```python
from build123d import *

# Parameters (mm, degrees)
SKETCH_1_W           = 30
SKETCH_1_H           = 48
EXTRUDE_1_DEPTH      = 2
SKETCH_2_R           = 1.6
CUT_EXTRUDE_1_DEPTH  = 2
SKETCH_3_R           = 8.75
CUT_EXTRUDE_2_DEPTH  = 2
SKETCH_4_W           = 30
SKETCH_4_H           = 2
EXTRUDE_2_DEPTH      = 17
SKETCH_14_W          = 0.5
SKETCH_14_H          = 2
CUT_EXTRUDE_6_DEPTH  = 67.738294854
SKETCH_15_W          = 2
SKETCH_15_H          = 65
EXTRUDE_7_DEPTH      = 50
SKETCH_16_W          = 5
SKETCH_16_H          = 65
EXTRUDE_8_DEPTH      = 35
SKETCH_17_R          = 2
CUT_EXTRUDE_7_DEPTH  = 35
SKETCH_18_W          = 2
SKETCH_18_H          = 28.264297395
EXTRUDE_9_DEPTH      = 1
EXTRUDE_10_REACH     = 87.675
SKETCH_19_W          = 2
SKETCH_19_H          = 19.264297395
CUT_EXTRUDE_8_DEPTH  = 6
CUT_EXTRUDE_9_DEPTH  = 6
CHAMFER_1_SIZE       = 1.5
SKETCH_22_R          = 1.5
SKETCH_22_W          = 4
SKETCH_22_H          = 11
CUT_EXTRUDE_10_DEPTH = 86.293610546


with BuildPart() as part:
    # Sketch 1 → Extrude 1 (new body)
    with BuildSketch(Plane.XY):
        Rectangle(SKETCH_1_W, SKETCH_1_H)
    extrude(amount=-EXTRUDE_1_DEPTH)

    # Sketch 2 → Cut-Extrude 1 (cut)
    with BuildSketch(Plane.XY):
        with Locations((-9.5, 19)):
            Circle(SKETCH_2_R)
        with Locations((9.5, 19)):
            Circle(SKETCH_2_R)
    extrude(amount=-CUT_EXTRUDE_1_DEPTH, mode=Mode.SUBTRACT)

    # Sketch 3 → Cut-Extrude 2 (cut)
    with BuildSketch(Plane.XY):
        with Locations((0, 13)):
            Circle(SKETCH_3_R)
    extrude(amount=-CUT_EXTRUDE_2_DEPTH, mode=Mode.SUBTRACT)

    # Sketch 4 → Extrude 2 (add)
    with BuildSketch(Plane(origin=(0, 24, 0), x_dir=(1, 0, 0), z_dir=(0, 1, 0))):
        with Locations((0, 1)):
            Rectangle(SKETCH_4_W, SKETCH_4_H)
    extrude(amount=EXTRUDE_2_DEPTH)

    # Sketch 14 → Cut-Extrude 6 (cut, through all)
    with BuildSketch(Plane.XZ.offset(24)):
        with Locations((-0.25, -1)):
            Rectangle(SKETCH_14_W, SKETCH_14_H)
    extrude(amount=-CUT_EXTRUDE_6_DEPTH, mode=Mode.SUBTRACT)


with BuildPart() as cut_extrude_6_piece_1:
    # of the separate pieces the step leaves, piece 1, a body of its own (cut_extrude_6_pieces)
    add(part.part.solids().sort_by_distance((15, -24, 0))[0])

    # Sketch 15 → Extrude 7 (add)
    with BuildSketch(Plane(origin=(15, 0, 0), x_dir=(0, 0, -1), z_dir=(1, 0, 0))):
        with Locations((1, 8.5)):
            Rectangle(SKETCH_15_W, SKETCH_15_H)
    extrude(amount=EXTRUDE_7_DEPTH)

    # Sketch 16 → Extrude 8 (add)
    with BuildSketch(Plane(origin=(0, 0, -2), x_dir=(-1, 0, 0), z_dir=(0, 0, -1))):
        with Locations((-62.5, 8.5)):
            Rectangle(SKETCH_16_W, SKETCH_16_H)
    extrude(amount=EXTRUDE_8_DEPTH)

    # Sketch 17 → Cut-Extrude 7 (cut)
    with BuildSketch(Plane(origin=(65, 0, 0), x_dir=(0, 0, -1), z_dir=(1, 0, 0))):
        with Locations(Location((13.5, 8.5, 0), (0, 0, 90))):
            Circle(SKETCH_17_R)
        with Locations(Location((23.5, 8.5, 0), (0, 0, 90))):
            Circle(SKETCH_17_R)
    extrude(amount=-CUT_EXTRUDE_7_DEPTH, mode=Mode.SUBTRACT)



with BuildPart() as cut_extrude_6_piece_2:
    # of the separate pieces the step leaves, piece 2, a body of its own (cut_extrude_6_pieces)
    add(part.part.solids().sort_by_distance((-15, -24, 0))[0])


with BuildPart() as cut_extrude_6_piece_1_1:
    add(cut_extrude_6_piece_1.part)

    add(cut_extrude_6_piece_2.part)  # Extrude 9 merges Cut-Extrude 6 piece 2
    # Sketch 18 → Extrude 9 (add)
    with BuildSketch(Plane(origin=(-0.5, 0, 0), x_dir=(0, 0, -1), z_dir=(1, 0, 0))):
        with Locations((1, -9.867851303)):
            Rectangle(SKETCH_18_W, SKETCH_18_H)
    extrude(amount=EXTRUDE_9_DEPTH)

    # Sketch 19 → Extrude 10 (add, up to next)
    with BuildSketch(Plane(origin=(-0.5, 0, 0), x_dir=(0, 0, -1), z_dir=(1, 0, 0)), mode=Mode.PRIVATE) as extrude_10_sk1:
        with Locations((1, 31.367851303)):
            Rectangle(SKETCH_19_W, SKETCH_19_H)
    extrude_10_tool1 = extrude(extrude_10_sk1.sketch, amount=EXTRUDE_10_REACH, mode=Mode.PRIVATE) - cut_extrude_6_piece_1_1.part
    add(extrude_10_tool1.solids().sort_by_distance((-0.5, 31.367851, -1))[0])

    # Sketch 20 → Cut-Extrude 8 (cut)
    with BuildSketch(Plane.XY):
        with BuildLine():
            Line((30, -5.5), (55, -5.5))
            ThreePointArc((55, -5.5), (58.5, -9), (55, -12.5))
            Line((55, -12.5), (30, -12.5))
            ThreePointArc((30, -12.5), (26.5, -9), (30, -5.5))
        make_face()
    extrude(amount=-CUT_EXTRUDE_8_DEPTH, mode=Mode.SUBTRACT)

    # Sketch 21 → Cut-Extrude 9 (cut)
    with BuildSketch(Plane(origin=(65, 0, 0), x_dir=(0, 0, -1), z_dir=(1, 0, 0))):
        with BuildLine():
            Line((7, -11), (32, -11))
            ThreePointArc((32, -11), (35, -14), (32, -17))
            Line((32, -17), (7, -17))
            ThreePointArc((7, -17), (4, -14), (7, -11))
        make_face()
    extrude(amount=-CUT_EXTRUDE_9_DEPTH, mode=Mode.SUBTRACT)

    # Chamfer 1
    chamfer_1_edges = [cut_extrude_6_piece_1_1.edges().sort_by_distance(p)[0] for p in [
        (60, 8.5, -2),
    ]]
    chamfer(chamfer_1_edges, length=CHAMFER_1_SIZE - 0.0001)  # a hair under: the kernel refuses the full size

    # Sketch 22 → Cut-Extrude 10 (cut, through all)
    with BuildSketch(Plane.XY):
        with Locations((-5, 38)):
            Circle(SKETCH_22_R)
        with Locations((-5, 27)):
            Circle(SKETCH_22_R)
        with Locations((7, 32.5)):
            Rectangle(SKETCH_22_W, SKETCH_22_H)
    extrude(amount=-CUT_EXTRUDE_10_DEPTH, mode=Mode.SUBTRACT)


solid = cut_extrude_6_piece_1_1.part
```
Work out the finished part from the listing and answer in its coordinate system (mm). A direction names the side the tool comes from. Round coordinates to 2 decimals unless told otherwise and drop trailing zeros. Loops run counter-clockwise (first coordinate to the right, second up) from the corner with the lowest first, then second, coordinate; pieces in that order, holes last.
(1) The part is cut by section A-A, the plane z = -18. Give the vertices of the cut face in (x, y), and give its area (3 significant figures).
Computed values:
outline: (60, -24) - (65, -24) - (65, -17) - (60, -17) - close; (60, -11) - (65, -11) - (65, 41) - (60, 41) - close
area: 295 mm2
(2) Find the intervals of material crossed by L1, parallel to Z at x = 63, y = 8; L2, parallel to Z at x = 63.25, y = 8.5; L3, parallel to X at y = 12, z = -25, in increasing order.
Computed values:
L1: z = -37 to -25.44, -21.56 to -15.44, -11.56 to 0
L2: z = -37 to -25.5, -21.5 to -15.5, -11.5 to 0
L3: x = 60 to 65
(3) The part is cut by section C-C, the plane z = -23.5. Give the vertices of the cut face in (x, y).
Computed values:
outline: (60, -24) - (65, -24) - (65, -17) - (60, -17) - close; (60, -11) - (65, -11) - (65, 6.5) - (60, 6.5) - close; (60, 10.5) - (65, 10.5) - (65, 41) - (60, 41) - close
(4) The part is cut by section B-B, the plane x = 38. Give the vertices of the cut face in (y, z), and give its area (3 significant figures).
Computed values:
outline: (-24, -2) - (-12.5, -2) - (-12.5, 0) - (-24, 0) - close; (-5.5, -2) - (41, -2) - (41, 0) - (-5.5, 0) - close
area: 116 mm2
(5) For faces 1 (the cylindrical face through (63, -14, -35)), 2 (the flat face through (-15, 8, -1)), 3 (the flat face through (63, 9, -37)), 4 (the cylindrical face through (-8.748, 13.185, -0.986)), 5 (the flat face through (21, 8, -2)), determine the directions among +Z, -Z, +X, -X, +Y, -Y from which every point of the face is accessible in a straight line to the end or side of a thin tool.
Computed values:
face 1: +X, -X
face 2: +Z, -Z, -X, +Y, -Y
face 3: -Z, +X, -X, +Y, -Y
face 4: +Z, -Z
face 5: -Z, -X, +Y, -Y
(6) The mould has two halves that part along Y. Classify faces 6 (the flat face through (7, 27, -1)), 7 (the flat face through (40, 41, -1)), 8 (the flat face through (60, 8, -20)): pulls with the +Y half, pulls with the -Y half, needs draft (parallel to the pull), parting line crosses it, or undercut.
Computed values:
face 6: undercut
face 7: pulls with the +Y half
face 8: needs draft
(7) The part is cut by section D-D, the plane y = 19. Give the vertices of the cut face in (x, z).
Computed values:
outline: (-15, -2) - (-11.1, -2) - (-11.1, 0) - (-15, 0) - close; (-7.9, -2) - (-6.37, -2) - (-6.37, 0) - (-7.9, 0) - close; (6.37, -2) - (7.9, -2) - (7.9, 0) - (6.37, 0) - close; (11.1, -2) - (58.5, -2) - (60, -3.5) - (60, -37) - (65, -37) - (65, 0) - (11.1, 0) - close
(8) Each of these flat-tipped pins is pushed along its axis until it touches: P1, Ø4, axis at x = 34, y = 14.5, coming from the -Z side; P2, Ø6, axis at x = 17.5, z = -4, coming from the +Y side. Where does it stop, or does it pass through?
Computed values:
P1: stops at z = -2
P2: stops at y = 41
